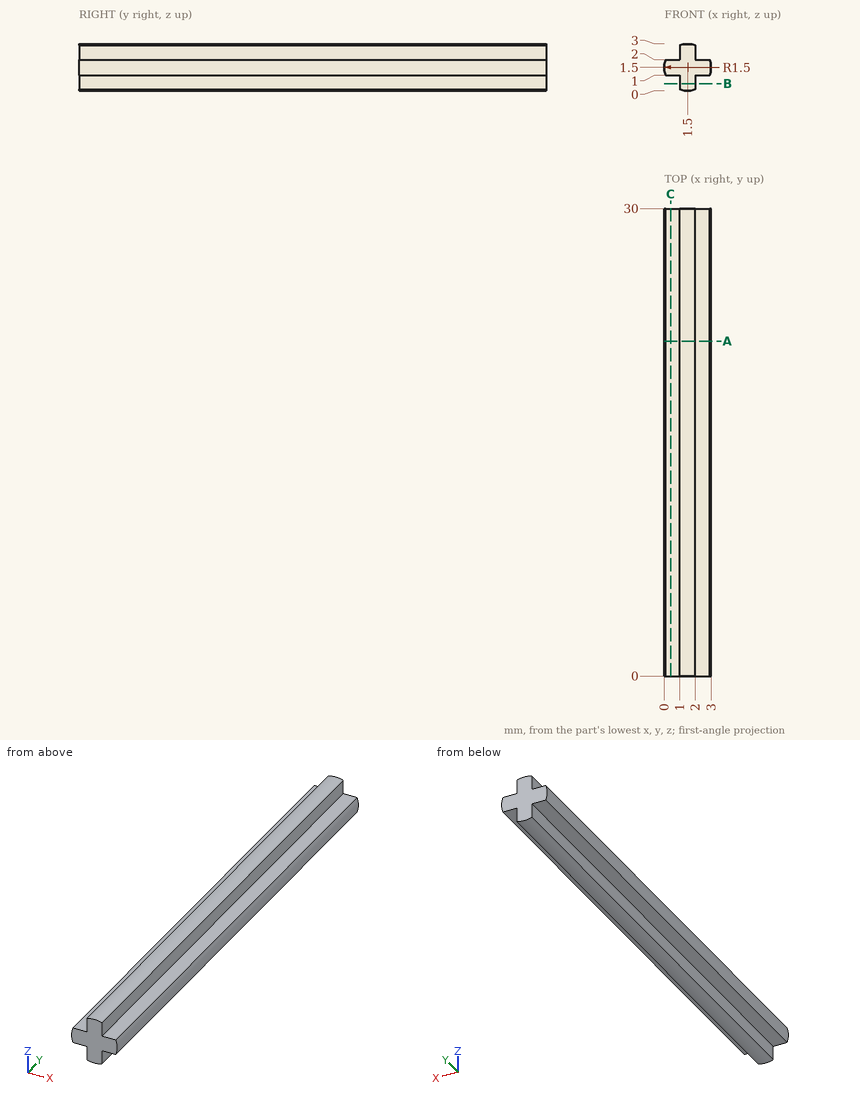
Study the drawing (mm; zero at the part's minimum x, y, z) and answer. Give positions to 0.01 mm unless a question says otherwise; leave off trailing zeros. Order: outer loops, then holes, each group sorted by start corner. A loop starts at its lowest first (then second) coordinate and runs counter-clockwise, first axis right, second up. Notation, with made-up numbers: (-39.75, -18) -> (-14.75, -18) arc R13 ccw to (-14.75, -2) -> close; hole circle Ø6 at (53.5, -24). An arc over 180 degrees is marked (long way). Write item = value, one per line.
1. Straight lines are drawn through the part: line 1 along X through (y, z) = (5.5, 2.1); line 2 along Z through (x, y) = (1.6, 20.75). For each, find the intervals that lie inside material, in ascending order.
Numbers:
line_1 = 1 to 2
line_2 = 0 to 3
2. A cutting plane is placed at B-B, the plane z = 0.45. Write down the section's boundary in (x, y).
Numbers:
outline = (1, 0) -> (2, 0) -> (2, 30) -> (1, 30) -> close
3. A cutting plane is placed at A-A, the plane y = 21.5. Write down the section's boundary in (x, z).
Numbers:
outline = (0.09, 1) -> (1, 1) -> (1, 0.09) arc R1.5 ccw to (2, 0.09) -> (2, 1) -> (2.91, 1) arc R1.5 ccw to (2.91, 2) -> (2, 2) -> (2, 2.91) arc R1.5 ccw to (1, 2.91) -> (1, 2) -> (0.09, 2) arc R1.5 ccw to start
4. A cutting plane is placed at C-C, the plane x = 0.4. Write down the section's boundary in (y, z).
Numbers:
outline = (0, 1) -> (30, 1) -> (30, 2) -> (0, 2) -> close
5. Given pin 1 (0.7 mm diameter, centred on y = 12, z = 0.5, fed in from +X); pin 2 (0.5 mm diameter, centred on y = 16, z = 2.5, fed in from -X); pin 3 (0.7 mm diameter, centred on x = 0.5, y = 12.5, fed in from -Z), each flat-ended and moving along its own axis, determine where each tip first touches the part or whether it passes through.
Numbers:
pin_1 = 2
pin_2 = 1
pin_3 = 1
